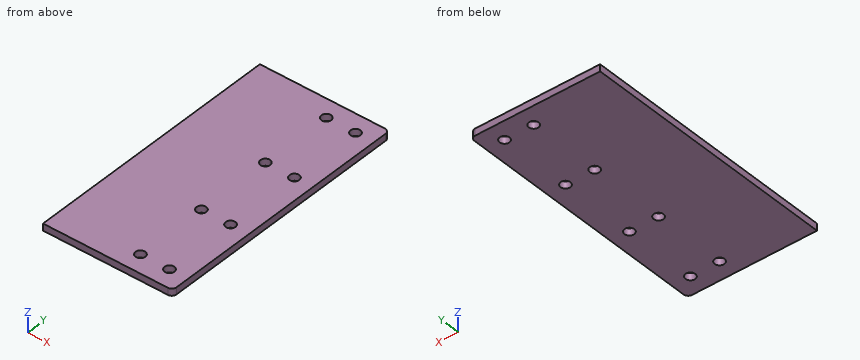
from build123d import *

# Parameters (mm, degrees)
F0_R     = 6.731
F1_DEPTH = 9.525


with BuildPart() as f1:
    # F0 (on Top) → F1 (new body)
    with BuildSketch(Plane.XY):
        with BuildLine():
            Line((-88.9, 177.8), (-88.9, -177.8))
            Line((-88.9, -177.8), (82.55, -177.8))
            ThreePointArc((82.55, -177.8), (87.040128, -175.940128), (88.9, -171.45))
            Line((88.9, -171.45), (88.9, 171.45))
            ThreePointArc((88.9, 171.45), (87.040128, 175.940128), (82.55, 177.8))
            Line((82.55, 177.8), (-88.9, 177.8))
        make_face()
        with Locations((23.50008, -152.4)):
            Circle(F0_R, mode=Mode.SUBTRACT)
        with Locations((63.5, -152.4)):
            Circle(F0_R, mode=Mode.SUBTRACT)
        with Locations((23.50008, -52.4002)):
            Circle(F0_R, mode=Mode.SUBTRACT)
        with Locations((63.5, -52.4002)):
            Circle(F0_R, mode=Mode.SUBTRACT)
        with Locations((23.50008, 52.4002)):
            Circle(F0_R, mode=Mode.SUBTRACT)
        with Locations((63.5, 52.4002)):
            Circle(F0_R, mode=Mode.SUBTRACT)
        with Locations((23.50008, 152.4)):
            Circle(F0_R, mode=Mode.SUBTRACT)
        with Locations((63.5, 152.4)):
            Circle(F0_R, mode=Mode.SUBTRACT)
    extrude(amount=F1_DEPTH)


solid = f1.part
Read the model definition and answer for the solid it produces. Units are mm, in the model's axes. Round coordinates to 2 decimals unless told otherwise and drop trailing zeros. Write each loop counter-clockwise with the first axis right and the second up, starting at its lowest first coordinate (ties: lowest second). Pieces come first, ordered by that corner, then holes.
Q1. Find section B-B on y = -152.4. Determine the outline of the cut face in (x, z) (3 decimals).
Values:
outline: (-88.9, 0) - (16.769, 0) - (16.769, 9.525) - (-88.9, 9.525) - close; (30.231, 0) - (56.769, 0) - (56.769, 9.525) - (30.231, 9.525) - close; (70.231, 0) - (88.9, 0) - (88.9, 9.525) - (70.231, 9.525) - close
Q2. Find section C-C on z = 7.5. State how many separate pieces and enclosed holes the cut face has, and give its area (3 significant figures).
Values:
separate pieces: 1
enclosed holes: 8
area: 62,100 mm2
Q3. Find section A-A on x = 63.5. Determine the outline of the cut face in (y, z) (3 decimals).
Values:
outline: (-177.8, 0) - (-159.131, 0) - (-159.131, 9.525) - (-177.8, 9.525) - close; (-145.669, 0) - (-59.131, 0) - (-59.131, 9.525) - (-145.669, 9.525) - close; (-45.669, 0) - (45.669, 0) - (45.669, 9.525) - (-45.669, 9.525) - close; (59.131, 0) - (145.669, 0) - (145.669, 9.525) - (59.131, 9.525) - close; (159.131, 0) - (177.8, 0) - (177.8, 9.525) - (159.131, 9.525) - close
Q4. Straight lines are drawn through the part: line 1 (Y direction, x = 63.5, z = 7.5); line 2 (Y direction, x = 28.5, z = 4); line 3 (X direction, y = -55, z = 2). For each, find the intervals that lie inside material, in ascending order.
Values:
line 1: y = -177.8 to -159.13, -145.67 to -59.13, -45.67 to 45.67, 59.13 to 145.67, 159.13 to 177.8
line 2: y = -177.8 to -156.91, -147.89 to -56.91, -47.89 to 47.89, 56.91 to 147.89, 156.91 to 177.8
line 3: x = -88.9 to 17.29, 29.71 to 57.29, 69.71 to 88.9
Q5. A flat-ended cylindrical pin translates along its axis: P1, Ø11, axis at x = 23.5, y = 52.4, coming from the +Z side. Find the tip coordinate at first contact, or state that the pin passes through.
Values:
P1: passes through
